The model under review builds one solid part; all positions refer to its coordinate system, in mm. A direction names the side the tool comes from. Coordinates: 2 decimals unless noted, no trailing zeros. Write each loop counter-clockwise with the first axis right and the second up, starting at its lowest first coordinate (ties: lowest second). Pieces come first, ordered by that corner, then holes. Notation, with made-up numbers: M 11.25,42.5 L 41.25,42.5 A9 cw 41.25,48.5 Z; hole C 64,86 d2. An arc over 180 degrees is marked long. Answer as a JSON object with one key per item and string values.
```python
from build123d import *

# Parameters (mm, degrees)
BOSS_EXTRUDE5_DEPTH  = 2.5
BOSS_EXTRUDE6_DEPTH  = 5
BOSS_EXTRUDE10_DEPTH = 10
CUT_EXTRUDE2_DEPTH   = 139.087836629
FILLET2_R            = 20


with BuildPart() as part:
    # Sketch3 → Boss-Extrude5 (new body)
    with BuildSketch(Plane.XY):
        with BuildLine():
            ThreePointArc((0, 1.975), (1.396535893, 1.396535893), (1.975, 0))
            Line((1.975, 0), (12.5, 0))
            ThreePointArc((12.5, 0), (8.838834765, 8.838834765), (0, 12.5))
            Line((0, 12.5), (0, 1.975))
        make_face()
        with BuildLine():
            Line((12.5, 0), (1.975, 0))
            ThreePointArc((1.975, 0), (1.396535893, -1.396535893), (0, -1.975))
            Line((0, -1.975), (0, -12.5))
            ThreePointArc((0, -12.5), (8.838834765, -8.838834765), (12.5, 0))
        make_face()
        with BuildLine():
            ThreePointArc((0, -1.975), (-1.396535893, -1.396535893), (-1.975, 0))
            Line((-1.975, 0), (-12.5, 0))
            ThreePointArc((-12.5, 0), (-8.838834765, -8.838834765), (0, -12.5))
            Line((0, -12.5), (0, -1.975))
        make_face()
        with BuildLine():
            Line((-12.5, 0), (-1.975, 0))
            ThreePointArc((-1.975, 0), (-1.396535893, 1.396535893), (0, 1.975))
            Line((0, 1.975), (0, 12.5))
            ThreePointArc((0, 12.5), (-8.838834765, 8.838834765), (-12.5, 0))
        make_face()
    extrude(amount=BOSS_EXTRUDE5_DEPTH)

    # Sketch5 → Boss-Extrude6 (add)
    with BuildSketch(Plane.XY.offset(2.5)):
        Polygon((-5, -134.975), (-5, -4.975), (0, -4.975), (5, -4.975), (5, -134.975), align=None)
    extrude(amount=BOSS_EXTRUDE6_DEPTH)

    # Sketch13 → Boss-Extrude10 (add)
    with BuildSketch(Plane(origin=(5, 0, 0), x_dir=(0, 0, -1), z_dir=(1, 0, 0))):
        Polygon((-7.5, -134.975), (-17.5, -134.975), (-17.5, -121.403681616), (-7.5, -121.403681616), (-2.5, -121.403681616), (7.5, -121.403681616), (7.5, -134.975), (-2.5, -134.975), align=None)
    extrude(amount=BOSS_EXTRUDE10_DEPTH)

    # Sketch14 → Cut-Extrude2 (cut, through all)
    with BuildSketch(Plane(origin=(0, 0, -7.5), x_dir=(-1, 0, 0), z_dir=(0, 0, -1))):
        with BuildLine():
            Line((-15, -134.975), (-15, -121.403681616))
            Line((-15, -121.403681616), (-5.003644464, -121.4036816))
            ThreePointArc((-5.003644464, -121.4036816), (-7.772477519, -129.831430515), (-15, -134.975))
        make_face()
    extrude(amount=-CUT_EXTRUDE2_DEPTH, mode=Mode.SUBTRACT)

    # Fillet2
    fillet2_edges = [part.edges().sort_by_distance(p)[0] for p in [
        (-5, -134.975, 5),
    ]]
    fillet(fillet2_edges, radius=FILLET2_R - 0.0001)  # a hair under: the kernel refuses the full size


solid = part.part
```
(1) Add section A-A on x = 10.75. Give the boundary of the cut face in (y, z).
Results list:
{"outline": "M -134.52,-7.5 L -132.82,-7.5 L -132.82,17.5 L -134.52,17.5 Z; M -6.38,0 L 6.38,0 L 6.38,2.5 L -6.38,2.5 Z"}
(2) Add section C-C on y = -31. Give the boundary of the cut face in (x, z), and give its area (3 significant figures).
Results list:
{"outline": "M -5,2.5 L 5,2.5 L 5,7.5 L -5,7.5 Z", "area": "50.0 mm²"}
(3) For faces 1 (the face through (0, -4.975, 5)), 2 (the face through (5, -127, -3)), 3 (the face through (5, -127, 12)), 4 (the face through (0, -3, 0)), list the 3-axis set-ups (+Z, -Z, +X, -X, +Y, -Y) from which the entire face can be reached by the end or side of a thin tool; tool diameter is ignored.
Results list:
{"face 1": "+Z, +X, -X, +Y", "face 2": "-Z, -X, -Y", "face 3": "+Z, -X, +Y, -Y", "face 4": "-Z, +X, -X, +Y"}
(4) Wall thickness on line 1 along Z through (x, y) = (2.75, -20); line 2 along Y through (x, z) = (8, 4); line 3 along Y through (x, z) = (12, -2.5): over which ranges is each line inside the solid? List them lowest first. Write a range as from..to.
Results list:
{"line 1": "2.5..7.5", "line 2": "-133.71..-130.13", "line 3": "-134.75..-133.65"}
(5) For pin 1 Ø1.5 at (y, z) = (-38, 5) entering from -X; pin 2 Ø5 at (x, z) = (6.5, -4) entering from +Y; pin 3 Ø7.5 at (x, y) = (5, 3) entering from -Z; pin 4 Ø3 at (x, y) = (-7.5, -21) entering from -Z, all flat-tipped, find the tip position at first contact; note any pin that passes through.
Results list:
{"pin 1": "x = -5", "pin 2": "y = -121.4", "pin 3": "z = 0", "pin 4": "through"}
(6) Draft analysis for pull direction X (two halves, no side actions). For faces 5 (the face through (-5, -61, 5)), 6 (the face through (8, -131, 17.5)), 7 (the face through (7.7, -129.73, 4.82)), state which applies: released by +X, released by -X, zero draft, split by the parting line, or undercut.
Results list:
{"face 5": "released by -X", "face 6": "zero draft", "face 7": "released by +X"}
